Geometry check sheet. Reference: the model listing, model coordinates, mm. Give positions to 0.01 mm unless a question says otherwise; leave off trailing zeros. Order: outer loops, then holes, each group sorted by start corner. A loop starts at its lowest first (then second) coordinate and runs counter-clockwise, first axis right, second up.
```python
from build123d import *

# Parameters (mm, degrees)
SKETCH_1_R               = 25
SKETCH_1_R_2             = 1.25
EXTRUDE_1_DEPTH          = 2.5
CUT_EXTRUDE_2_DEPTH      = 36.443617197
CUT_EXTRUDE_2_DEPTH_BACK = 36.443617197
SKETCH_3_R               = 1
SKETCH_3_R_2             = 4
CUT_EXTRUDE_5_DEPTH      = 10
FILLET_2_R               = 3


with BuildPart() as part:
    # 草图1 → 凸台-拉伸1 (new body)
    with BuildSketch(Plane.XY):
        Circle(SKETCH_1_R)
        with Locations((0, 22)):
            Circle(SKETCH_1_R_2, mode=Mode.SUBTRACT)
        with Locations((22, 0)):
            Circle(SKETCH_1_R_2, mode=Mode.SUBTRACT)
        with Locations((0, -22)):
            Circle(SKETCH_1_R_2, mode=Mode.SUBTRACT)
        with Locations(Location((-22, 0, 0), (0, 0, 180))):
            Circle(SKETCH_1_R_2, mode=Mode.SUBTRACT)
    extrude(amount=EXTRUDE_1_DEPTH)

    # 草图3 → 切除-拉伸2 (cut, two sides: drawn at the far end of the back side and taken through both)
    with BuildSketch(Plane(origin=(0, 0, 0), x_dir=(-1, 0, 0), z_dir=(0, 0, -1)).offset(-CUT_EXTRUDE_2_DEPTH_BACK)):
        with Locations((0, 6.2)):
            Circle(SKETCH_3_R)
        Circle(SKETCH_3_R_2)
        with Locations((0, -6.2)):
            Circle(SKETCH_3_R)
    extrude(amount=CUT_EXTRUDE_2_DEPTH + CUT_EXTRUDE_2_DEPTH_BACK, mode=Mode.SUBTRACT)

    # 草图5 → 切除-拉伸5 (cut)
    with BuildSketch(Plane(origin=(0, 0, 0), x_dir=(-1, 0, 0), z_dir=(0, 0, -1))):
        with BuildLine():
            ThreePointArc((-2.638187412, 24.860409634), (-17.67766953, 17.67766953), (-24.860409634, 2.638187412))
            ThreePointArc((-24.860409634, 2.638187412), (-10.606601718, 10.606601718), (-2.638187412, 24.860409634))
        make_face()
        with BuildLine():
            ThreePointArc((-2.638187412, -24.860409634), (-10.606601718, -10.606601718), (-24.860409634, -2.638187412))
            ThreePointArc((-24.860409634, -2.638187412), (-17.67766953, -17.67766953), (-2.638187412, -24.860409634))
        make_face()
        with BuildLine():
            ThreePointArc((24.860409634, -2.638187412), (10.606601718, -10.606601718), (2.638187412, -24.860409634))
            ThreePointArc((2.638187412, -24.860409634), (17.67766953, -17.67766953), (24.860409634, -2.638187412))
        make_face()
        with BuildLine():
            ThreePointArc((24.860409634, 2.638187412), (17.67766953, 17.67766953), (2.638187412, 24.860409634))
            ThreePointArc((2.638187412, 24.860409634), (10.606601718, 10.606601718), (24.860409634, 2.638187412))
        make_face()
    extrude(amount=-CUT_EXTRUDE_5_DEPTH, mode=Mode.SUBTRACT)

    # 圆角2
    fillet_2_edges = [part.edges().sort_by_distance(p)[0] for p in [
        (2.638187412, 24.860409634, 1.25),
        (24.860409634, 2.638187412, 1.25),
        (24.860409634, -2.638187412, 1.25),
        (2.638187412, -24.860409634, 1.25),
        (-2.638187412, -24.860409634, 1.25),
        (-24.860409634, -2.638187412, 1.25),
        (-24.860409634, 2.638187412, 1.25),
        (-2.638187412, 24.860409634, 1.25),
    ]]
    fillet(fillet_2_edges, radius=FILLET_2_R)


solid = part.part
```
Q1. Cross-section at A-A, the plane x = -22. Record the boundary of the cut face in (y, z), and give its area (3 significant figures).
Q2. Release check for a two-part mould opening along Y. For faces 1 (the face through (10.751, 10.464, 1.232)), 2 (the face through (-10.751, -10.464, 1.232)), 3 (the face through (-0.27, -23.22, 1.23)) record: pulls with the +Y half, pulls with the -Y half, needs draft (parallel to the pull), parting line crosses it, or undercut.
Q3. Cross-section at D-D, the plane y = 11. Record the boundary of the cut face in (x, z).
Q4. Thickness scan on L1, parallel to Y at x = 0, z = 0.6; L2, parallel to Y at x = -22, z = 0.95; L3, parallel to Y at x = 2.5, z = 1.1. Record the ranges inside material, lowest first.
Q5. Gauge pin test, flat ends, axial feed: P1, Ø1.5, axis at y = 3, z = 0.5, coming from the -X side; P2, Ø6, axis at x = -6.5, y = -13, coming from the -Z side. Record the tip position at first contact, or that the pin passes through.
Q6. Cross-section at C-C, the plane z = 1.5. Give the number of separate pieces and of enclosed holes in the cut face, and give its area (3 significant figures).
Answers follow:
1. outline: (-3.47, 0) - (-1.25, 0) - (-1.25, 2.5) - (-3.47, 2.5) - close; (1.25, 0) - (3.47, 0) - (3.47, 2.5) - (1.25, 2.5) - close
1. area: 11.1 mm2
2. face 1: pulls with the +Y half
2. face 2: pulls with the -Y half
2. face 3: undercut
3. outline: (-10.22, 0) - (10.22, 0) - (10.22, 2.5) - (-10.22, 2.5) - close
4. L1: y = -25 to -23.25, -20.75 to -7.2, -5.2 to -4, 4 to 5.2, 7.2 to 20.75, 23.25 to 25
4. L2: y = -3.47 to -1.25, 1.25 to 3.47
4. L3: y = -24.05 to -3.12, 3.12 to 24.05
5. P1: stops at x = -24.29
5. P2: stops at z = 0
6. separate pieces: 1
6. enclosed holes: 7
6. area: 1,030 mm2
